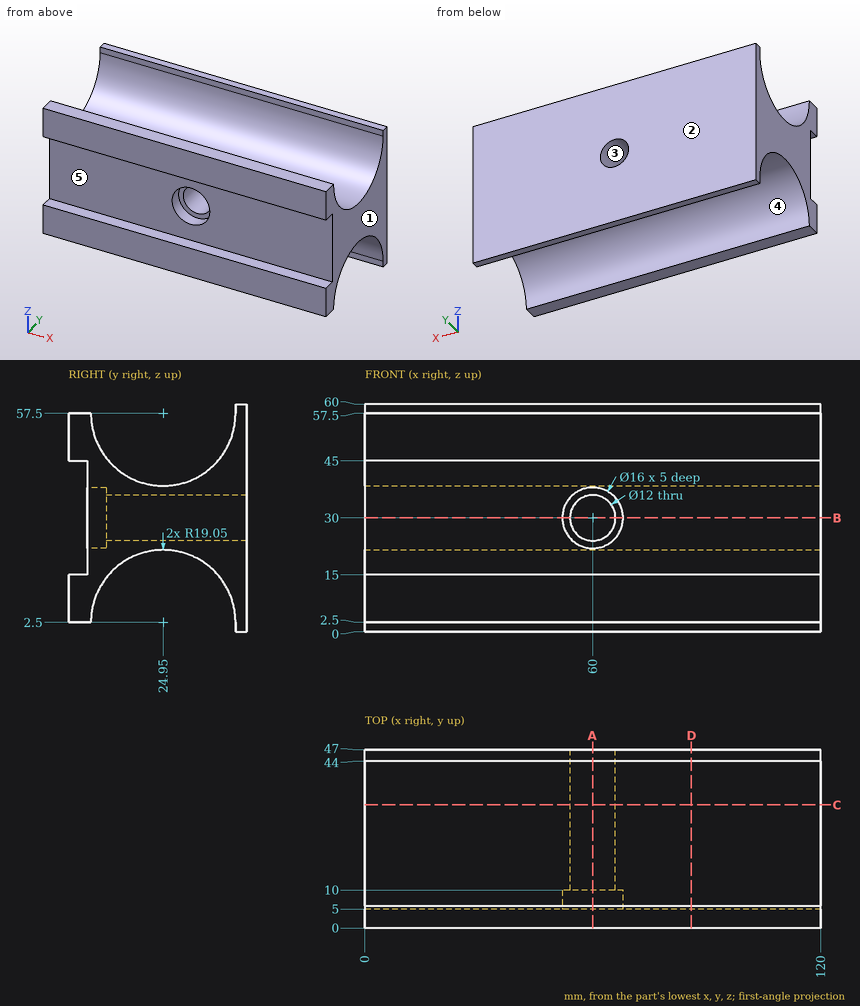
The figure shows three views and two pictorial views of one solid part (mm, origin at its lowest corner). Answer the questions. A direction names the side the tool comes from. Round coordinates to 2 decimals unless told otherwise and drop trailing zeros. Write each loop counter-clockwise with the first axis right and the second up, starting at its lowest first coordinate (ties: lowest second). Pieces come first, ordered by that corner, then holes. Notation, with made-up numbers: (9.5, 11.25) - (62.5, 11.25) arc R28 cw to (62.5, 35.25) - close; hole circle Ø8 at (-24, -11). An arc over 180 degrees is marked (long way). Answer in a Markdown table with one row per item. Add a question column.
1. A cutting plane is placed at C-C, the plane y = 32.5. Determine the outline of the cut face in (x, z).
2. For the marked faces 4 and 5, determine the directions among +Z, -Z, +X, -X, +Y, -Y from which every point of the face is accessible in a straight line to the end or side of a thin tool.
3. The mould has two halves that part along X. Classify the marked faces 1, 2 and 3: +X half, -X half, draft (parallel to the pull), parting line (faces both ways), or undercut.
4. A cutting plane is placed at B-B, the plane z = 30. Determine the outline of the cut face in (x, y).
5. A cutting plane is placed at D-D, the plane x = 86. Determine the outline of the cut face in (y, z), and give its area (3 significant figures).
6. Given pin 1 (5.5 mm diameter, centred on x = 58.5, y = 3.5, fed in from +Z); pin 2 (0.8 mm diameter, centred on x = 58, z = 1, fed in from -Y); pin 3 (3 mm diameter, centred on x = 71, y = 2, fed in from -Z); pin 4 (7 mm diameter, centred on x = 60, z = 30, fed in from +Y), each flat-ended and moving along its own axis, determine where each tip first touches the part or whether it passes through.
7. Find the intervals of material crossed by line 1 along Y through (x, z) = (22, 30); line 2 along Y through (x, z) = (80.5, 46); line 3 along Y through (x, z) = (96, 41.5), in increasing order. Write a range as from..to.
8. A cutting plane is placed at A-A, the plane x = 60. Determine the outline of the cut face in (y, z).
Worked out:
| question | item | result |
|---|---|---|
| 1 | outline | (0, 19.99) - (120, 19.99) - (120, 40.01) - (0, 40.01) - close; hole circle Ø12 at (60, 30) |
| 2 | face 4 | -Z, +X, -X |
| 2 | face 5 | +X, -X, -Y |
| 3 | face 1 | +X half |
| 3 | face 2 | draft |
| 3 | face 3 | undercut |
| 4 | outline | (0, 5) - (52, 5) - (52, 10) - (54, 10) - (54, 47) - (0, 47) - close; (66, 10) - (68, 10) - (68, 5) - (120, 5) - (120, 47) - (66, 47) - close |
| 5 | outline | (0, 2.5) - (5.9, 2.5) arc R19.05 cw to (44, 2.5) - (44, 0) - (47, 0) - (47, 60) - (44, 60) - (44, 57.5) arc R19.05 cw to (5.9, 57.5) - (0, 57.5) - (0, 45) - (5, 45) - (5, 15) - (0, 15) - close |
| 5 | area | 1,310 mm^2 |
| 6 | pin 1 | z = 57.5 |
| 6 | pin 2 | y = 44 |
| 6 | pin 3 | z = 2.5 |
| 6 | pin 4 | through |
| 7 | line 1 | 5..47 |
| 7 | line 2 | 0..9.76, 40.14..47 |
| 7 | line 3 | 5..14.61, 35.29..47 |
| 8 | outline | (0, 2.5) - (5.9, 2.5) arc R19.05 cw to (44, 2.5) - (44, 0) - (47, 0) - (47, 24) - (10, 24) - (10, 22) - (5, 22) - (5, 15) - (0, 15) - close; (0, 45) - (5, 45) - (5, 38) - (10, 38) - (10, 36) - (47, 36) - (47, 60) - (44, 60) - (44, 57.5) arc R19.05 cw to (5.9, 57.5) - (0, 57.5) - close |
